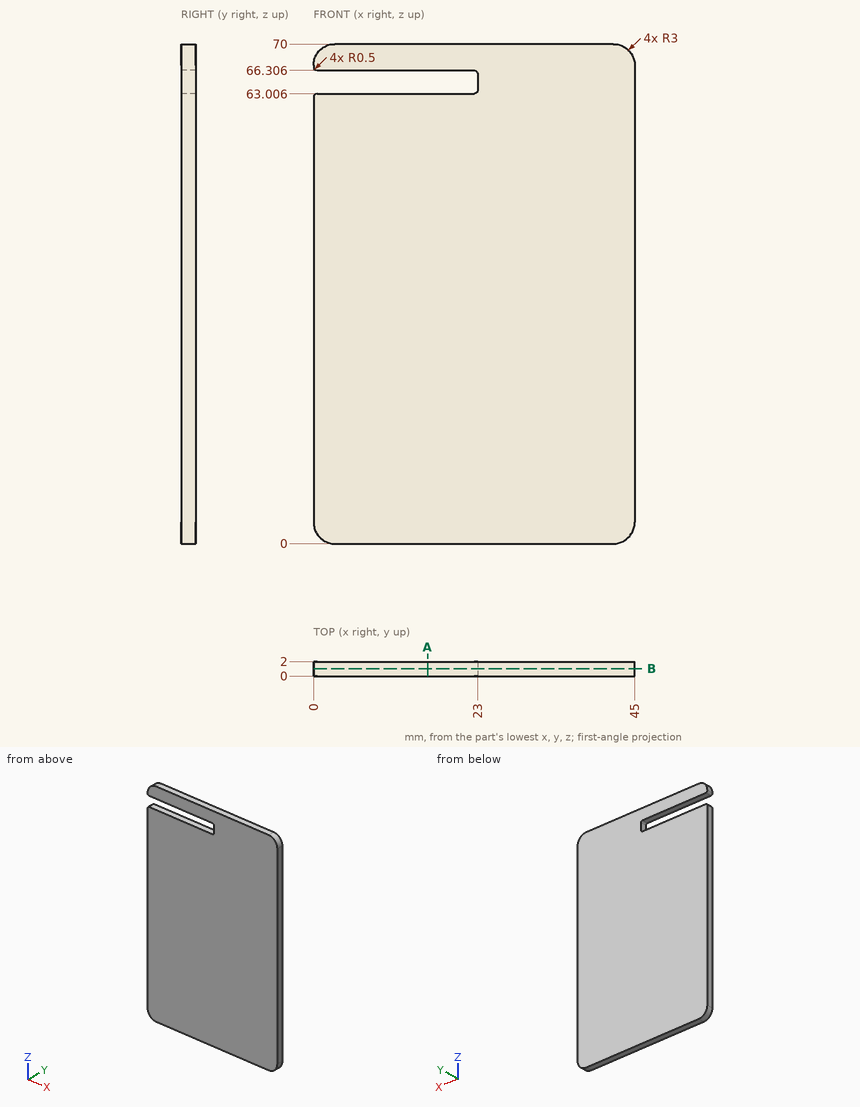
Could you check a few things on this drawing? It's one solid part, dimensions in mm from its lowest x, y, z. Coordinates: 2 decimals unless noted, no trailing zeros. Order: outer loops, then holes, each group sorted by start corner. A loop starts at its lowest first (then second) coordinate and runs counter-clockwise, first axis right, second up. Notation, with made-up numbers: M 49,16 L 56,16 A9 cw 56,21 Z; hole C 40,18 d2. An arc over 180 degrees is marked long. Use one line per item in the form item = value. Start each with the question number.
1. Suppose I cut it at B-B on y = 1.05. Write out the boundary of the cut face in (x, z), then the cut area to 3 significant figures.
2. Suppose I cut it at A-A on x = 16. Write out the boundary of the cut face in (y, z).
3. For pin 1 (1 mm diameter, centred on x = 14, y = 1.5, fed in from -Z), with a flat end and sliding along its axis, tell me the tip position at first contact or that it passes through.
4. Please list where these lines run through material, in increasing order: line 1 (Z direction, x = 18, y = 1); line 2 (Z direction, x = 2, y = 1.55); line 3 (X direction, y = 0.9, z = 66).
Geometry says:
q1.outline = M 0,3 A3 ccw 3,0 L 42,0 A3 ccw 45,3 L 45,67 A3 ccw 42,70 L 3,70 A3 ccw 0,67 L 0,66.81 A0.5 ccw 0.5,66.31 L 22.5,66.31 A0.5 cw 23,65.81 L 23,63.51 A0.5 cw 22.5,63.01 L 0.5,63.01 A0.5 ccw 0,62.51 Z
q1.area = 3,070 mm^2
q2.outline = M 0,0 L 2,0 L 2,63.01 L 0,63.01 Z; M 0,66.31 L 2,66.31 L 2,70 L 0,70 Z
q3.pin_1 = 0
q4.line_1 = 0 to 63.01, 66.31 to 70
q4.line_2 = 0.17 to 63.01, 66.31 to 69.83
q4.line_3 = 22.96 to 45
